Check sheet for the modelled part. Datum: model origin and axes. Units: mm. A direction names the side the tool comes from. Give positions to 0.01 mm unless a question says otherwise; leave off trailing zeros. Order: outer loops, then holes, each group sorted by start corner. A loop starts at its lowest first (then second) coordinate and runs counter-clockwise, first axis right, second up.
```python
from build123d import *

# Parameters (mm, degrees)
PAD015_DEPTH         = 9
SKETCH051_R          = 2.65
POCKET023_DEPTH      = 37.240539
POCKET023_DEPTH_BACK = 16.501
SKETCH052_R          = 2.65
POCKET024_DEPTH      = 25.001
POCKET024_DEPTH_BACK = 5.001
SKETCH053_R          = 4.5
POCKET025_DEPTH      = 31.240539
SKETCH055_R          = 2.15
POCKET026_DEPTH      = 30.001
POCKET031_DEPTH      = 20.001


with BuildPart() as part:
    # Sketch047 → Pad015 (new body, symmetric)
    with BuildSketch(Plane(origin=(0, 0, 0), x_dir=(-1, 0, 0), z_dir=(0, 1, 0))):
        with BuildLine():
            Line((-22.5, -16.5), (-20, -16.5))
            Line((-20, -16.5), (-20, 0))
            Line((-20, 0), (0, 0))
            Line((0, 0), (0, 6))
            Line((0, 6), (0, 37.239539))
            Line((-30, 37.239539), (0, 37.239539))
            Line((-30, 19.460461), (-30, 37.239539))
            Line((-30, 19.460461), (-26, 6))
            Line((-26, 6), (-26, -13))
            ThreePointArc((-26, -13), (-24.974874, -15.474874), (-22.5, -16.5))
        make_face()
    extrude(amount=PAD015_DEPTH, both=True)

    # Sketch051 → Pocket023 (cut, two sides)
    with BuildSketch(Plane(origin=(10, 0, 0), x_dir=(1, 0, 0), z_dir=(0, 0, 1))) as pocket023_sk:
        Circle(SKETCH051_R)
    extrude(amount=POCKET023_DEPTH, mode=Mode.SUBTRACT)
    extrude(pocket023_sk.sketch, amount=-POCKET023_DEPTH_BACK, mode=Mode.SUBTRACT)

    # Sketch052 → Pocket024 (cut, two sides)
    with BuildSketch(Plane(origin=(25, 0, -10), x_dir=(0, 1, 0), z_dir=(1, 0, 0))) as pocket024_sk:
        Circle(SKETCH052_R)
    extrude(amount=-POCKET024_DEPTH, mode=Mode.SUBTRACT)
    extrude(pocket024_sk.sketch, amount=POCKET024_DEPTH_BACK, mode=Mode.SUBTRACT)

    # Sketch053 → Pocket025 (cut, through all)
    with BuildSketch(Plane(origin=(10, 0, 6), x_dir=(1, 0, 0), z_dir=(0, 0, 1))):
        Circle(SKETCH053_R)
    extrude(amount=POCKET025_DEPTH, mode=Mode.SUBTRACT)

    # Sketch055 → Pocket026 (cut, through all)
    with BuildSketch(Plane(origin=(0, 0, 0), x_dir=(0, -1, 0), z_dir=(-1, 0, 0))):
        with Locations((0, 28.35)):
            Circle(SKETCH055_R)
    extrude(amount=-POCKET026_DEPTH, mode=Mode.SUBTRACT)

    # Sketch066 → Pocket031 (cut, through all)
    with BuildSketch(Plane(origin=(10, 0, 28.35), x_dir=(0, 1, 0), z_dir=(1, 0, 0))):
        Polygon((-7.778175, 0), (0, 7.778175), (7.778175, 0), (0, -7.778175), align=None)
    extrude(amount=POCKET031_DEPTH, mode=Mode.SUBTRACT)


solid = part.part
```
(1) Cross-section at B-B on x = 18.5. Enter the section's corners in (y, z).
Response values:
outline: (-9, 0) - (9, 0) - (9, 37.24) - (-9, 37.24) - close; hole (-7.78, 28.35) - (0, 20.57) - (7.78, 28.35) - (0, 36.13) - close
(2) Release check for a two-part mould opening along Z. For faces 1 (the face through (28.028, 0.126, 12.824)), 2 (the face through (15, 0, 37.24)), 3 (the face through (23.04, -0.57, -12.59)), 4 (the face through (19.86, -3.944, 32.185)) record: released by +Z, released by -Z, zero draft, split by the parting line, or undercut.
Response values:
face 1: released by -Z
face 2: released by +Z
face 3: undercut
face 4: undercut
(3) Gauge pin test, flat ends, axial feed: pin 1 Ø1 at (y, z) = (6, 28) entering from +X; pin 2 Ø1 at (y, z) = (3, -3) entering from -X; pin 3 Ø3 at (x, y) = (10, 0) entering from +Z; pin 4 Ø8.5 at (y, z) = (0, -10) entering from +X. Record the tip position at first contact, or that the pin passes through.
Response values:
pin 1: stops at x = 10
pin 2: stops at x = 20
pin 3: passes through
pin 4: stops at x = 26
(4) Cross-section at C-C on y = -3.5. Enter the section's corners in (x, z).
Response values:
outline: (0, 0) - (20, 0) - (20, -16.5) - (22.5, -16.5) arc R3.5 ccw to (26, -13) - (26, 6) - (30, 19.46) - (30, 24.07) - (12.83, 24.07) - (12.83, 6) - (7.17, 6) - (7.17, 37.24) - (0, 37.24) - close; (12.83, 32.63) - (30, 32.63) - (30, 37.24) - (12.83, 37.24) - close
(5) Cross-section at A-A on z = -10. Enter the section's corners in (x, y), then the cut area to 3 significant figures.
Response values:
outline: (20, -9) - (26, -9) - (26, -2.65) - (20, -2.65) - close; (20, 2.65) - (26, 2.65) - (26, 9) - (20, 9) - close
area: 76.2 mm2
(6) Set-up check for faces 5 (the face through (5.504, 0.198, 21.401)), 6 (the face through (21, 0, -16.5)), 7 (the face through (15, 9, 17)), 8 (the face through (12, -2, 0)), 9 (the face through (19.86, -3.835, 24.406)): record each of +Z, -Z, +X, -X, +Y, -Y from which the full face is reachable in a straight line by a thin tool's end or side.
Response values:
face 5: +Z
face 6: -Z, +X, -X, +Y, -Y
face 7: +Z, -Z, +X, -X, +Y
face 8: -Z, -X, +Y, -Y
face 9: +X
(7) Cross-section at D-D on z = 5. Enter the section's corners in (x, y), then the cut area to 3 significant figures.
Response values:
outline: (0, -9) - (26, -9) - (26, 9) - (0, 9) - close; hole circle Ø5.3 at (10, 0)
area: 446 mm2
(8) Material ranges on L1, parallel to Y at x = 24.25, z = -10; L2, parallel to Z at x = 5, y = 0; L3, parallel to Z at x = 3, y = -7, recorded low to high.
Response values:
L1: y = -9 to -2.65, 2.65 to 9
L2: z = 0 to 26.2, 30.5 to 37.24
L3: z = 0 to 37.24
